from build123d import *

# Parameters (mm, degrees)
PAD_DEPTH       = 60
POCKET_DEPTH    = 50
POCKET001_DEPTH = 408.7079232475
POCKET002_DEPTH = 408.4326470939


with BuildPart() as part:
    # Sketch → Pad (new body)
    with BuildSketch(Plane.XY):
        Polygon((450, 0), (450, 90), (356, 87.18), (355.64, 99.18), (343.64, 98.82), (344, 86.82), (6, 76.68), (5.64, 88.6800000001), (-6.36, 88.3200000001), (-6, 76.32), (-50, 75), (-50, 0), align=None)
    extrude(amount=PAD_DEPTH)

    # Sketch001 (on Face14 of Pad) → Pocket (cut)
    with BuildSketch(Plane.XY.offset(60)):
        Polygon((-50, 15), (-50, 74), (450, 74), (450, 0), (356, 2.82), (356.3, 12.82), (344.3, 13.18), (344, 3.18), (6, 13.32), (6.3, 23.32), (-5.7, 23.68), (-6, 13.68), align=None)
    extrude(amount=-POCKET_DEPTH, mode=Mode.SUBTRACT)

    # Sketch002 (on Face26 of Pocket) → Pocket001 (cut, through all)
    with BuildSketch(Plane(origin=(355.5953641722, -10.6678609252, 0), x_dir=(0.0299865091, 0.9995503035, 0), z_dir=(0.9995503035, -0.0299865091, 0))):
        with BuildLine():
            ThreePointArc((23.4984280855, 54), (19.9988591841, 55.4495689014), (21.4484280855, 51.95))
            ThreePointArc((21.4484280855, 51.95), (17.8329435114, 39), (21.4484280855, 26.05))
            ThreePointArc((21.4484280855, 26.05), (19.9988591841, 22.5504310986), (23.4984280855, 24))
            Line((23.4984280855, 24), (23.4984280855, 54))
        make_face()
    extrude(amount=-POCKET001_DEPTH, mode=Mode.SUBTRACT)

    # Sketch003 (on Face14 of Pocket001) → Pocket002 (cut, through all)
    with BuildSketch(Plane(origin=(358.2929363573, 10.7487880907, 0), x_dir=(-0.0299865091, 0.9995503035, 0), z_dir=(0.9995503035, 0.0299865091, 0))):
        with BuildLine():
            ThreePointArc((88.470997005, 54), (84.9714281036, 55.4495689014), (86.420997005, 51.95))
            ThreePointArc((86.420997005, 51.95), (82.8055124309, 39), (86.420997005, 26.05))
            ThreePointArc((86.420997005, 26.05), (84.9714281036, 22.5504310986), (88.470997005, 24))
            Line((88.470997005, 24), (88.470997005, 54))
        make_face()
    extrude(amount=-POCKET002_DEPTH, mode=Mode.SUBTRACT)


solid = part.part
Work out the finished part from the listing and answer in its coordinate system (mm). A direction names the side the tool comes from. Round coordinates to 2 decimals unless told otherwise and drop trailing zeros. Write each loop counter-clockwise with the first axis right and the second up, starting at its lowest first coordinate (ties: lowest second). Pieces come first, ordered by that corner, then holes. Notation, with made-up numbers: (15, 39) - (34, 39) arc R23 cw to (34, 48) - close; hole circle Ø5 at (-4, -5). An arc over 180 degrees is marked (long way). Answer in a Markdown table with one row per item. Add a question column.
1. A cutting plane is placed at C-C, the plane z = 5.5. Determine the outline of the cut face in (x, y), and give its area (3 significant figures).
2. A cutting plane is placed at A-A, the plane z = 38.5. Determine the outline of the cut face in (x, y), and give its area (3 significant figures).
3. A cutting plane is placed at B-B, the plane x = 236. Determine the outline of the cut face in (y, z), and give its area (3 significant figures).
4. For faces 1 (the cylindrical face through (350.214, 7.335, 39.191)), 2 (the cylindrical face through (349.89, 93.34, 39.19)), 3 (the flat face through (197, 74, 35)), 4 (the flat face through (450, 64.4, 9.6)), determine the directions among +Z, -Z, +X, -X, +Y, -Y from which every point of the face is accessible in a straight line to the end or side of a thin tool.
5. Given pin 1 (1 mm diameter, centred on x = 319.5, y = 12, fed in from +Z); pin 2 (2 mm diameter, centred on y = 82.5, z = 13.5, fed in from -X); pin 3 (2 mm diameter, centred on y = 17, z = 47, fed in from +X), each flat-ended and moving along its own axis, determine where each tip first touches the part or whether it passes through.
6. Find the intervals of material crossed by line 1 along Y through (x, z) = (406.5, 9.5) (3 decimals); line 2 along Z through (x, y) = (67, 70.5); line 3 along Y through (x, z) = (266, 18.5), in increasing order. Write a range as from..to.
7. A cutting plane is placed at D-D, the plane y = 55.5. Determine the outline of the cut face in (x, z).
Worked out:
| question | item | result |
|---|---|---|
| 1 | outline | (-50, 0) - (450, 0) - (450, 90) - (356, 87.18) - (355.64, 99.18) - (343.64, 98.82) - (344, 86.82) - (6, 76.68) - (5.64, 88.68) - (-6.36, 88.32) - (-6, 76.32) - (-50, 75) - close |
| 1 | area | 41,500 mm^2 |
| 2 | outline | (-50, 0) - (450, 0) - (356, 2.82) - (356.13, 7.16) - (344.13, 7.52) - (344, 3.18) - (6, 13.32) - (6.13, 17.66) - (-5.87, 18.02) - (-6, 13.68) - (-50, 15) - close; (-50, 74) - (450, 74) - (450, 90) - (356, 87.18) - (355.81, 93.52) - (343.81, 93.16) - (344, 86.82) - (6, 76.68) - (5.81, 83.02) - (-6.19, 82.66) - (-6, 76.32) - (-50, 75) - close |
| 2 | area | 8,260 mm^2 |
| 3 | outline | (0, 0) - (83.58, 0) - (83.58, 60) - (74, 60) - (74, 10) - (6.42, 10) - (6.42, 60) - (0, 60) - close |
| 3 | area | 1,640 mm^2 |
| 4 | face 1 | +X |
| 4 | face 2 | -X, +Y |
| 4 | face 3 | +Z, +X, -X |
| 4 | face 4 | +Z, -Z, +X, +Y, -Y |
| 5 | pin 1 | z = 10 |
| 5 | pin 2 | x = -6.22 |
| 5 | pin 3 | x = 6.14 |
| 6 | line 1 | 0..88.695 |
| 6 | line 2 | 0..10 |
| 6 | line 3 | 0..5.52, 74..84.48 |
| 7 | outline | (-50, 0) - (450, 0) - (450, 10) - (-50, 10) - close |
